Can you work these out from the model? Positions are in its coordinate system, mm. A direction names the side the tool comes from. Coordinates: 2 decimals unless noted, no trailing zeros. Order: outer loops, then holes, each group sorted by start corner. A loop starts at its lowest first (then second) coordinate and runs counter-clockwise, first axis right, second up. Notation, with made-up numbers: (57, -20) - (70, -20) arc R35 cw to (70, 19) - close; hole circle Ø6 at (-0.5, 87). An arc over 180 degrees is marked (long way). Use a Markdown table: item, result. Add a question column.
(1) I want a section at B-B (z = 1.5). List the corners of the cut face in (x, y) for me, and give its area (3 significant figures).
(2) We'd pull the mould along X, two halves only. Please class faces 4 (the cylindrical face through (0, 10, 0)), 5 (the cylindrical face through (4.5, 6.3, 0.1)), 6 (the cylindrical face through (12.54, 2.46, 1.05)), 7 (the cylindrical face through (-7.46, 2.46, 1.05)): pulls with the +X half, pulls with the -X half, needs draft (parallel to the pull), parting line crosses it, or undercut.
(3) On a 3-axis mill with a long thin cutter (end or side, diameter ignored), from which of +Z, -Z, +X, -X, +Y, -Y can I reach the whole of each face in a straight line? I mean faces 1 (the cylindrical face through (-4.5, 6.3, -0.1)), 2 (the flat face through (-12.3, 0, -1.8)), 3 (the flat face through (12.4, 5, -1.8)). Say none if no direction works.
(4) I want a section at D-D (z = 6). List the corners of the cut face in (x, y) for me, and give its area (3 significant figures).
(5) If I drill on L1, parallel to Z at x = 10, y = 2.7; L2, parallel to X at y = 2, z = 0; L3, parallel to Y at x = 6, z = 1.5, over which ranges is the centre line in solid material (lowest first)? Write a range as [from, to].
(6) I want a section at C-C (y = 4.25). List the corners of the cut face in (x, z) for me.
(7) I want a section at A-A (y = 2.5). List the corners of the cut face in (x, z) for me.
(8) For pin 1 Ø1.5 at (y, z) = (3, -5.5) entering from -X; pin 2 Ø5 at (x, z) = (0, -6) entering from -Y, each with a flat end and sliding along its axis, tell me the tip position at first contact or that it passes through.
```python
from build123d import *

# Parameters (mm, degrees)
BOSS_EXTRUDE1_DEPTH = 9.5
SKETCH1_3_R         = 2.75
BOSS_EXTRUDE2_DEPTH = 5
CUT_EXTRUDE2_DEPTH  = 16
SKETCH7_R           = 0.5
BOSS_EXTRUDE3_DEPTH = 0.5


with BuildPart() as part:
    # Sketch1 → Boss-Extrude1 (new body)
    with BuildSketch(Plane(origin=(0, 0, 0), x_dir=(1, 0, 0), z_dir=(0, 1, 0))):
        with BuildLine():
            Line((8.08, 7.5), (-8.08, 7.5))
            Line((-8.08, 7.5), (-8.08, 5.153988747))
            ThreePointArc((-8.08, 5.153988747), (-4.5, 0), (-8.08, -5.153988747))
            Line((-8.08, -5.153988747), (-8.08, -7.5))
            Line((-8.08, -7.5), (8.08, -7.5))
            Line((8.08, -7.5), (8.08, -5.153988747))
            ThreePointArc((8.08, -5.153988747), (4.5, 0), (8.08, 5.153988747))
            Line((8.08, 5.153988747), (8.08, 7.5))
        make_face()
    extrude(amount=BOSS_EXTRUDE1_DEPTH)

    # Sketch1_3 → Boss-Extrude2 (add)
    with BuildSketch(Plane(origin=(0, 0, 0), x_dir=(1, 0, 0), z_dir=(0, 1, 0))):
        with BuildLine():
            Line((-8.08, 5.153988747), (-8.08, 7.5))
            Line((-8.08, 7.5), (-10, 7.5))
            ThreePointArc((-10, 7.5), (-17.5, 0), (-10, -7.5))
            Line((-10, -7.5), (-8.08, -7.5))
            Line((-8.08, -7.5), (-8.08, -5.153988747))
            ThreePointArc((-8.08, -5.153988747), (-4.5, 0), (-8.08, 5.153988747))
        make_face()
        with Locations((-10, 0)):
            Circle(SKETCH1_3_R, mode=Mode.SUBTRACT)
        with BuildLine():
            Line((10, 7.5), (8.08, 7.5))
            Line((8.08, 7.5), (8.08, 5.153988747))
            ThreePointArc((8.08, 5.153988747), (4.5, 0), (8.08, -5.153988747))
            Line((8.08, -5.153988747), (8.08, -7.5))
            Line((8.08, -7.5), (10, -7.5))
            ThreePointArc((10, -7.5), (17.5, 0), (10, 7.5))
        make_face()
        with Locations((10, 0)):
            Circle(SKETCH1_3_R, mode=Mode.SUBTRACT)
    extrude(amount=BOSS_EXTRUDE2_DEPTH)

    # Sketch3 → Cut-Extrude2 (cut, through all)
    with BuildSketch(Plane.XY.offset(7.5)):
        with BuildLine():
            Line((1.6e-08, 9.5), (-8.08, 9.5))
            Line((-8.08, 9.5), (-8.08, 5))
            ThreePointArc((-8.08, 5), (-4.624294534, 8.299133313), (1.6e-08, 9.5))
        make_face()
        with BuildLine():
            Line((8.08, 9.5), (1.6e-08, 9.5))
            ThreePointArc((1.6e-08, 9.5), (4.624294548, 8.299133305), (8.08, 5))
            Line((8.08, 5), (8.08, 9.5))
        make_face()
        with BuildLine():
            ThreePointArc((-3.97617907, 0), (-0.503818326, -5.06892702), (4.1, -1))
            ThreePointArc((4.1, -1), (4.06892702, -0.496181674), (3.97617907, 0))
            Line((3.97617907, 0), (-3.97617907, 0))
        make_face()
        with BuildLine():
            Line((-3.97617907, 0), (3.97617907, 0))
            ThreePointArc((3.97617907, 0), (0, 3.1), (-3.97617907, 0))
        make_face()
    extrude(amount=-CUT_EXTRUDE2_DEPTH, mode=Mode.SUBTRACT)

    # Sketch7 → Boss-Extrude3 (add, symmetric)
    with BuildSketch(Plane.XY):
        with Locations((0, 9.5)):
            Circle(SKETCH7_R)
    extrude(amount=BOSS_EXTRUDE3_DEPTH, both=True)


solid = part.part
```
Answers follow:
| question | item | result |
|---|---|---|
| 1 | outline | (-17.35, 0) - (-12.3, 0) - (-12.3, 5) - (-17.35, 5) - close; (-7.7, 0) - (-3.98, 0) arc R4.1 cw to (3.98, 0) - (7.7, 0) - (7.7, 5) - (4.71, 5) - (4.71, 8.25) arc R9.5 ccw to (-4.71, 8.25) - (-4.71, 5) - (-7.7, 5) - close; (12.3, 0) - (17.35, 0) - (17.35, 5) - (12.3, 5) - close |
| 1 | area | 148 mm² |
| 2 | face 4 | parting line crosses it |
| 2 | face 5 | pulls with the +X half |
| 2 | face 6 | undercut |
| 2 | face 7 | undercut |
| 3 | face 1 | -X, +Y |
| 3 | face 2 | +Z, -Z, +X, -X, -Y |
| 3 | face 3 | +X, +Y |
| 4 | outline | (-14.5, 0) - (-3.98, 0) arc R4.1 cw to (3.98, 0) - (14.5, 0) - (14.5, 5) - (8.08, 5) arc R9.5 ccw to (-8.08, 5) - (-14.5, 5) - close |
| 4 | area | 178 mm² |
| 5 | L1 | z = [-7.5, -2.75], [2.75, 7.5] |
| 5 | L2 | x = [-17.5, -12.75], [-7.25, -2.79], [2.79, 7.25], [12.75, 17.5] |
| 5 | L3 | y = [0, 5] |
| 6 | outline | (-10, -7.5) - (10, -7.5) arc R7.5 ccw to (10, 7.5) - (-10, 7.5) arc R7.5 ccw to start; hole circle Ø5.5 at (-10, 0); hole circle Ø5.5 at (10, 0) |
| 7 | outline | (-10, -7.5) - (-2.14, -7.5) - (-2.14, 7.5) - (-10, 7.5) arc R7.5 ccw to start; (2.14, -7.5) - (10, -7.5) arc R7.5 ccw to (10, 7.5) - (2.14, 7.5) - close; hole circle Ø5.5 at (-10, 0); hole circle Ø5.5 at (10, 0) |
| 8 | pin 1 | stops at x = -15.8 |
| 8 | pin 2 | stops at y = 2.25 |
